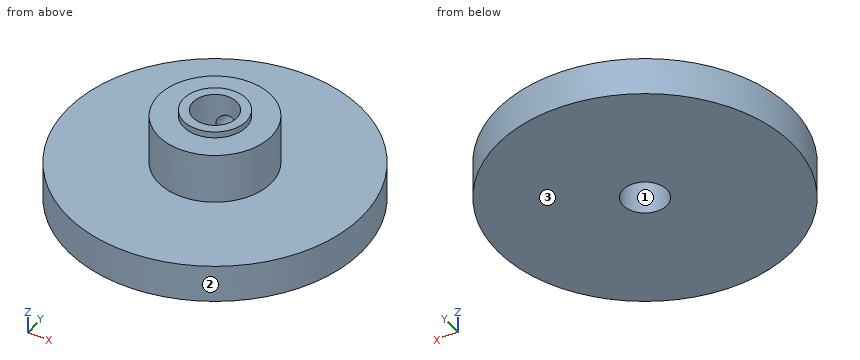
```python
from build123d import *

# Parameters (mm, degrees)
SKETCH_1_R          = 23.5
EXTRUDE_1_DEPTH     = 6
SKETCH_2_R          = 9
EXTRUDE_2_DEPTH     = 8
SKETCH_3_R          = 3.5
CUT_EXTRUDE_1_DEPTH = 37.062445841
SKETCH_4_R          = 1.75
CUT_EXTRUDE_2_DEPTH = 37.062445841
EXTRUDE_START       = 1
SKETCH_5_R          = 5
SKETCH_5_R_2        = 3.5
EXTRUDE_3_DEPTH     = 1


with BuildPart() as part:
    # 草图1 → 凸台-拉伸1 (new body)
    with BuildSketch(Plane.XY):
        Circle(SKETCH_1_R)
    extrude(amount=EXTRUDE_1_DEPTH)

    # 草图2 → 凸台-拉伸2 (add)
    with BuildSketch(Plane.XY.offset(6)):
        Circle(SKETCH_2_R)
    extrude(amount=EXTRUDE_2_DEPTH)

    # 草图3 → 切除-拉伸1 (cut, through all)
    with BuildSketch(Plane.XY.offset(14)):
        Circle(SKETCH_3_R)
    extrude(amount=-CUT_EXTRUDE_1_DEPTH, mode=Mode.SUBTRACT)

    # 草图4 → 切除-拉伸2 (cut, through all)
    with BuildSketch(Plane(origin=(0, 0, 0), x_dir=(1, 0, 0), z_dir=(0, 1, 0))):
        with Locations(Location((0, -10, 0), (0, 0, 90))):
            Circle(SKETCH_4_R)
    extrude(amount=CUT_EXTRUDE_2_DEPTH, mode=Mode.SUBTRACT)

    # 草图5 → 凸台-拉伸3 (add)
    with BuildSketch(Plane.XY.offset(14).offset(EXTRUDE_START)):
        Circle(SKETCH_5_R)
        Circle(SKETCH_5_R_2, mode=Mode.SUBTRACT)
    extrude(amount=-EXTRUDE_3_DEPTH)


solid = part.part
```
CAD build for the part. Positions are in the model's coordinates, mm. Face numbers are marked on the shaded views. Round coordinates to 2 decimals unless told otherwise and drop trailing zeros. Write each loop counter-clockwise with the first axis right and the second up, starting at its lowest first coordinate (ties: lowest second). Pieces come first, ordered by that corner, then holes. Notation, with made-up numbers: (-21.5, -25.75) -> (8.5, -25.75) arc R10 cw to (8.5, -9.75) -> close; hole circle Ø4 at (-19.5, -25). An arc over 180 degrees is marked (long way). Answer in a Markdown table with one row per item. Add a question column.
Item 1: Saw through at B-B, the plane y = -1. Write the cut outline in (x, z).
Item 2: Saw through at C-C, the plane z = 5. Write the cut outline in (x, y).
Item 3: Saw through at D-D, the plane x = 8. Write the cut outline in (y, z).
Item 4: Saw through at A-A, the plane x = 0. Write the cut outline in (y, z), then the cut area to 3 significant figures.
Item 5: Drill centre lines: line 1 (Y direction, x = 0, z = 10); line 2 (Z direction, x = 3, y = 8); line 3 (Z direction, x = 13, y = 3.5). Where is each one in solid material? Low to high. Write a range as from..to.
Item 6: Mould opens along Y. For the marked faces 1, 2 and 3 say: pulls with the +Y half, pulls with the -Y half, needs draft (parallel to the pull), parting line crosses it, or undercut.
Item 7: Drop flat-ended pins along their axis: pin 1 Ø4 at (x, z) = (0, 10) entering from +Y; pin 2 Ø2 at (x, y) = (-4.5, -17) entering from +Z; pin 3 Ø4 at (x, y) = (0, 0) entering from +Z; pin 4 Ø1 at (x, z) = (-0.5, 2.5) entering from -Y. Give the stop position or say it passes through.
Findings below:
| question | item | result |
|---|---|---|
| 1 | outline | (-23.48, 0) -> (-3.35, 0) -> (-3.35, 15) -> (-4.9, 15) -> (-4.9, 14) -> (-8.94, 14) -> (-8.94, 6) -> (-23.48, 6) -> close; (3.35, 0) -> (23.48, 0) -> (23.48, 6) -> (8.94, 6) -> (8.94, 14) -> (4.9, 14) -> (4.9, 15) -> (3.35, 15) -> close |
| 2 | outline | circle Ø47 at (0, 0); hole circle Ø7 at (0, 0) |
| 3 | outline | (-22.1, 0) -> (22.1, 0) -> (22.1, 6) -> (4.12, 6) -> (4.12, 14) -> (-4.12, 14) -> (-4.12, 6) -> (-22.1, 6) -> close |
| 4 | outline | (-23.5, 0) -> (-3.5, 0) -> (-3.5, 15) -> (-5, 15) -> (-5, 14) -> (-9, 14) -> (-9, 6) -> (-23.5, 6) -> close; (3.5, 0) -> (23.5, 0) -> (23.5, 6) -> (9, 6) -> (9, 8.25) -> (3.5, 8.25) -> close; (3.5, 11.75) -> (9, 11.75) -> (9, 14) -> (5, 14) -> (5, 15) -> (3.5, 15) -> close |
| 4 | area | 312 mm^2 |
| 5 | line 1 | y = -9..-3.5 |
| 5 | line 2 | z = 0..14 |
| 5 | line 3 | z = 0..6 |
| 6 | face 1 | undercut |
| 6 | face 2 | parting line crosses it |
| 6 | face 3 | needs draft |
| 7 | pin 1 | stops at y = 9 |
| 7 | pin 2 | stops at z = 6 |
| 7 | pin 3 | passes through |
| 7 | pin 4 | stops at y = -23.5 |
